Work out the finished part from the listing and answer in its coordinate system (mm). Face numbers are marked on the shaded views. A direction names the side the tool comes from. Round coordinates to 2 decimals unless told otherwise and drop trailing zeros. Write each loop counter-clockwise with the first axis right and the second up, starting at its lowest first coordinate (ties: lowest second). Pieces come first, ordered by that corner, then holes. Notation, with made-up numbers: (7.5, 7.25) - (63.5, 7.25) arc R26 cw to (63.5, 28.25) - close; hole circle Ø3 at (26, -11). An arc over 180 degrees is marked (long way). Write item = value, one per line. Start each with the question number.
from build123d import *

# Parameters (mm, degrees)
SKETCH_W      = 10
SKETCH_H      = 171
PAD_DEPTH     = 8
SKETCH001_R   = 20.5
PAD001_DEPTH  = 5
PAD002_DEPTH  = 40
SKETCH004_R   = 1.7
HOLE_DEPTH    = 40.001
PAD003_DEPTH  = 3
SKETCH006_R   = 1.75
SKETCH006_R_2 = 4
POCKET_DEPTH  = 40.001


with BuildPart() as part:
    # Sketch → Pad (new body)
    with BuildSketch(Plane.XY):
        with Locations((67.5, 135.5)):
            Rectangle(SKETCH_W, SKETCH_H)
    extrude(amount=-PAD_DEPTH)

    # Sketch001 → Pad001 (join)
    with BuildSketch(Plane.XY):
        with Locations((67.5, 50)):
            Circle(SKETCH001_R)
    extrude(amount=-PAD001_DEPTH)

    # Sketch003 → Pad002 (join)
    with BuildSketch(Plane.XY):
        with BuildLine():
            Line((50, 221), (85, 221))
            Line((85, 221), (85, 233.13051))
            ThreePointArc((85, 233.13051), (84.908676, 233.599521), (84.648047, 234))
            Line((84.648047, 234), (73.398047, 245.61949))
            ThreePointArc((73.398047, 245.61949), (72.987667, 245.900948), (72.5, 246))
            Line((72.5, 246), (62.5, 246))
            ThreePointArc((62.5, 246), (62.012333, 245.900948), (61.601953, 245.61949))
            Line((61.601953, 245.61949), (50.351953, 234))
            ThreePointArc((50.351953, 234), (50.091324, 233.599521), (50, 233.13051))
            Line((50, 233.13051), (50, 221))
        make_face()
    extrude(amount=-PAD002_DEPTH)

    # Sketch004 → Hole (cut, through all)
    with BuildSketch(Plane.XY):
        with Locations((57.5, 226)):
            Circle(SKETCH004_R)
        with Locations((77.5, 226)):
            Circle(SKETCH004_R)
        with Locations((75, 236)):
            Circle(SKETCH004_R)
        with Locations((60, 236)):
            Circle(SKETCH004_R)
    extrude(amount=-HOLE_DEPTH, mode=Mode.SUBTRACT)

    # Sketch005 → Pad003 (join)
    with BuildSketch(Plane.XY):
        with BuildLine():
            Line((55, 167.87868), (55, 102.12132))
            ThreePointArc((55, 102.12132), (55.62132, 100.62132), (57.12132, 100))
            Line((57.12132, 100), (77.87868, 100))
            ThreePointArc((77.87868, 100), (79.37868, 100.62132), (80, 102.12132))
            Line((80, 102.12132), (80, 167.87868))
            ThreePointArc((80, 167.87868), (79.37868, 169.37868), (77.87868, 170))
            Line((77.87868, 170), (57.12132, 170))
            ThreePointArc((57.12132, 170), (55.62132, 169.37868), (55, 167.87868))
        make_face()
    extrude(amount=-PAD003_DEPTH)

    # Sketch006 → Pocket (cut, through all)
    with BuildSketch(Plane.XY):
        with Locations((79.344039, 38.155961)):
            Circle(SKETCH006_R)
        with Locations((79.344039, 61.844039)):
            Circle(SKETCH006_R)
        with Locations((55.655961, 61.844039)):
            Circle(SKETCH006_R)
        with Locations((55.655961, 38.155961)):
            Circle(SKETCH006_R)
        with Locations((67.5, 50)):
            Circle(SKETCH006_R_2)
    extrude(amount=-POCKET_DEPTH, mode=Mode.SUBTRACT)


solid = part.part
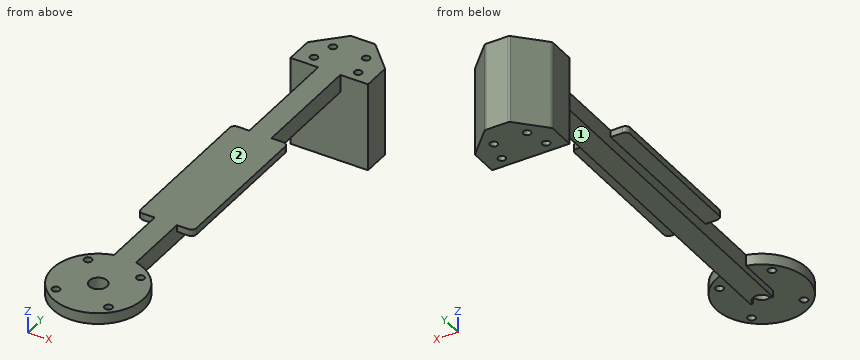
1. Consider line 1 (X direction, y = 226, z = -16); line 2 (X direction, y = 50, z = -1); line 3 (X direction, y = 171, z = -7.5). Determine where each line is inside the solid, lowest interval first.
2. Find section B-B on z = -23. Give the vertices of the cut face in (x, y).
3. Find section A-A on x = 67.5. Give the vertices of the cut face in (y, z).
4. Which of the six approach directions +Z, -Z, +X, -X, +Y, -Y give full straight-line access (tool end or side, diameter ignored) to the marked faces 1 and 2?
5. Find section D-D on y = 230. Give the vertices of the cut face in (x, z), plus the area to 3 significant figures.
6. Each of these flat-tipped pins is pushed along its axis until it touches: pin 1 (8.5 mm diameter, centred on x = 58, y = 145, fed in from -Z); pin 2 (1.5 mm diameter, centred on x = 76.5, z = -1.5, fed in from +Y); pin 3 (3 mm diameter, centred on x = 57.5, y = 226, fed in from +Z); pin 4 (8.5 mm diameter, centred on x = 75.5, y = 132.5, fed in from -Z). Where does it stop, or does it pass through?
7. Find section C-C on y = 165. Give the vertices of the cut face in (x, z).
Answer key:
q1.line_1 = 50 to 55.8, 59.2 to 75.8, 79.2 to 85
q1.line_2 = 47 to 63.5, 71.5 to 88
q1.line_3 = 62.5 to 72.5
q2.outline = (50, 221) - (85, 221) - (85, 233.13) arc R1.25 ccw to (84.65, 234) - (73.4, 245.62) arc R1.25 ccw to (72.5, 246) - (62.5, 246) arc R1.25 ccw to (61.6, 245.62) - (50.35, 234) arc R1.25 ccw to (50, 233.13) - close; hole circle Ø3.4 at (57.5, 226); hole circle Ø3.4 at (60, 236); hole circle Ø3.4 at (75, 236); hole circle Ø3.4 at (77.5, 226)
q3.outline = (29.5, -5) - (46, -5) - (46, 0) - (29.5, 0) - close; (54, -8) - (221, -8) - (221, -40) - (246, -40) - (246, 0) - (54, 0) - close
q4.face_1 = -Z, +X, -X, -Y
q4.face_2 = +Z, +X, -X, +Y, -Y
q5.outline = (50, -40) - (85, -40) - (85, 0) - (50, 0) - close
q5.area = 1,400 mm²
q6.pin_1 = -3
q6.pin_2 = 243.19
q6.pin_3 = through
q6.pin_4 = -8
q7.outline = (55, -3) - (62.5, -3) - (62.5, -8) - (72.5, -8) - (72.5, -3) - (80, -3) - (80, 0) - (55, 0) - close
